Here's how the part is built. I have some questions about the finished solid (model axes, mm). Face numbers are marked on the shaded views. A direction names the side the tool comes from. Round coordinates to 2 decimals unless told otherwise and drop trailing zeros. Write each loop counter-clockwise with the first axis right and the second up, starting at its lowest first coordinate (ties: lowest second). Pieces come first, ordered by that corner, then holes. Notation, with made-up numbers: M 44,28.5 L 60,28.5 A32 cw 60,55.5 Z; hole C -13,-9.75 d4. An arc over 180 degrees is marked long. Use one line per item in the form item = value. Start each with the question number.
Q1. We'd pull the mould along Y, two halves only. Please class the marked faces 3, 4, 5 and 6: +Y half, -Y half, draft (parallel to the pull), parting line (faces both ways), or undercut.
Q2. I'm going to push flat-ended pins straight in: pin 1 Ø4 at (x, y) = (35.95, 15.88) entering from +Z; pin 2 Ø5 at (y, z) = (12, 2) entering from +X; pin 3 Ø4 at (y, z) = (14.5, -1.5) entering from -X; pin 4 Ø1.8 at (y, z) = (16.5, -1) entering from +X. Where does each tip first touch, or does it pass through?
Q3. I want a section at B-B on x = 20.5. List the corners of the cut face in (y, z) for me.
Q4. I want a section at C-C on z = 1.5. List the corners of the cut face in (x, y) for me (3 decimals).
Q5. I want a section at A-A on z = -1.5. List the corners of the cut face in (x, y) for me (3 decimals), and give its area (3 significant figures).
Q6. I need wall thicknesses on line 1 along Z through (x, y) = (11, 14); line 2 along X through (y, z) = (16, 1); line 3 along X through (y, z) = (16.5, 4). Which ranges of each line are inside material? Lowest first, please. Write a range as from..to.
Q7. For the marked faces 1 and 2, which set-ups out of +Z, -Z, +X, -X, +Y, -Y let a thin tool reach every point of the face, with its end or its side?
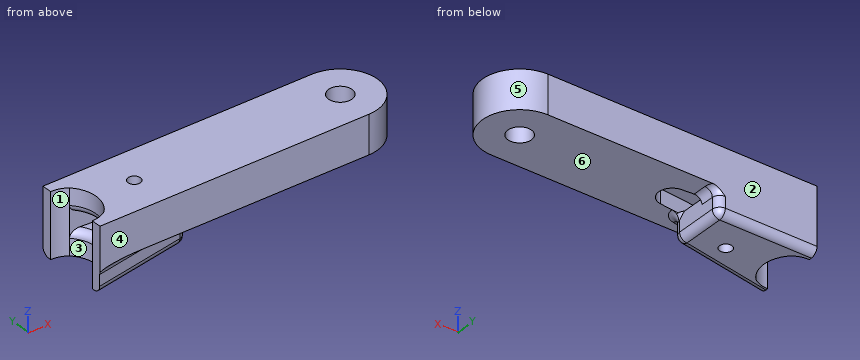
```python
from build123d import *

# Parameters (mm, degrees)
EXTRUDE_1_DEPTH     = 2.2
SKETCH_2_W          = 36.5
SKETCH_2_H          = 10.05
EXTRUDE_2_DEPTH     = 3.25
SKETCH_3_W          = 36.5
SKETCH_3_H          = 10.05
EXTRUDE_3_DEPTH     = 3.25
CUT_EXTRUDE_1_DEPTH = 30
SKETCH_6_R          = 5.025
EXTRUDE_4_DEPTH     = 8.7
SKETCH_8_R          = 1.675
SKETCH_8_R_2        = 0.84
CUT_EXTRUDE_3_DEPTH = 55
SKETCH_9_W          = 53.416465659
SKETCH_9_H          = 14.532409192
CUT_EXTRUDE_4_DEPTH = 3.5
SKETCH_10_R         = 1.6
CUT_EXTRUDE_5_DEPTH = 10
CUT_EXTRUDE_6_DEPTH = 3.5
FILLET_1_R          = 1
FILLET_2_R          = 1
FILLET_3_R          = 1


with BuildPart() as part:
    # 草图1 → 凸台-拉伸1 (new body)
    with BuildSketch(Plane.XY):
        with BuildLine():
            Line((1.539836705, 12.851012384), (15.55297303, 14.251012384))
            ThreePointArc((15.55297303, 14.251012384), (17.193415997, 16.063512384), (15.55297303, 17.876012384))
            Line((15.55297303, 17.876012384), (1.500532553, 18.901012384))
            ThreePointArc((1.500532553, 18.901012384), (0.527100583, 19.384612538), (-0.54702697, 19.551012384))
            Line((-0.54702697, 19.551012384), (-0.54702697, 20.901012384))
            Line((-0.54702697, 20.901012384), (19.51277613, 20.901012384))
            Line((19.51277613, 20.901012384), (35.95297303, 20.901012384))
            Line((35.95297303, 20.901012384), (35.95297303, 10.851012384))
            Line((35.95297303, 10.851012384), (-0.54702697, 10.851012384))
            Line((-0.54702697, 10.851012384), (-0.54702697, 12.201012384))
            ThreePointArc((-0.54702697, 12.201012384), (0.54584768, 12.367273294), (1.539836705, 12.851012384))
        make_face()
    extrude(amount=EXTRUDE_1_DEPTH)

    # 草图2 → 凸台-拉伸2 (add)
    with BuildSketch(Plane(origin=(0, 0, 0), x_dir=(-1, 0, 0), z_dir=(0, 0, -1))):
        with Locations((-17.70297303, 15.876012384)):
            Rectangle(SKETCH_2_W, SKETCH_2_H)
    extrude(amount=EXTRUDE_2_DEPTH)

    # 草图3 → 凸台-拉伸3 (add)
    with BuildSketch(Plane.XY.offset(2.2)):
        with Locations((17.70297303, 15.876012384)):
            Rectangle(SKETCH_3_W, SKETCH_3_H)
    extrude(amount=EXTRUDE_3_DEPTH)

    # 草图4 → 切除-拉伸1 (cut, symmetric)
    with BuildSketch(Plane.XY):
        with BuildLine():
            Line((-0.54702697, 19.551012384), (-2.235397712, 16.616091152))
            Line((-2.235397712, 16.616091152), (-1.110896638, 12.310548833))
            Line((-1.110896638, 12.310548833), (-0.54702697, 12.201012384))
            ThreePointArc((-0.54702697, 12.201012384), (0.54584768, 12.367273294), (1.539836705, 12.851012384))
            ThreePointArc((1.539836705, 12.851012384), (2.773180655, 15.88415254), (1.500532553, 18.901012384))
            ThreePointArc((1.500532553, 18.901012384), (0.527100583, 19.384612538), (-0.54702697, 19.551012384))
        make_face()
    extrude(amount=CUT_EXTRUDE_1_DEPTH, both=True, mode=Mode.SUBTRACT)

    # 草图6 → 凸台-拉伸4 (add)
    with BuildSketch(Plane(origin=(0, 0, -3.25), x_dir=(-1, 0, 0), z_dir=(0, 0, -1))):
        with Locations((-35.95297303, 15.876012384)):
            Circle(SKETCH_6_R)
    extrude(amount=-EXTRUDE_4_DEPTH)

    # 草图8 → 切除-拉伸3 (cut)
    with BuildSketch(Plane(origin=(0, 0, -3.25), x_dir=(-1, 0, 0), z_dir=(0, 0, -1))):
        with Locations((-49.45297303, 15.876012384)):
            Circle(SKETCH_8_R)
        with Locations(Location((-7.95297303, 15.856360308, 0), (0, 0, 180))):
            Circle(SKETCH_8_R_2)
    extrude(amount=-CUT_EXTRUDE_3_DEPTH, mode=Mode.SUBTRACT)

    # 草图9 → 切除-拉伸4 (cut)
    with BuildSketch(Plane(origin=(0, 0, -3.25), x_dir=(-1, 0, 0), z_dir=(0, 0, -1))):
        with Locations((-39.607660409, 15.039406696)):
            Rectangle(SKETCH_9_W, SKETCH_9_H)
    extrude(amount=-CUT_EXTRUDE_4_DEPTH, mode=Mode.SUBTRACT)

    # 草图10 → 切除-拉伸5 (cut)
    with BuildSketch(Plane.XY.offset(5.45)):
        with Locations((35.95297303, 15.876012384)):
            Circle(SKETCH_10_R)
    extrude(amount=-CUT_EXTRUDE_5_DEPTH, mode=Mode.SUBTRACT)

    # 草图11 → 切除-拉伸6 (cut)
    with BuildSketch(Plane(origin=(0, 0, -3.25), x_dir=(-1, 0, 0), z_dir=(0, 0, -1))):
        Polygon((-12.89942758, 13.294850275), (0.782882432, 10.851012384), (0, 8.730799831), (-15.448021962, 9.415407398), align=None)
    extrude(amount=-CUT_EXTRUDE_6_DEPTH, mode=Mode.SUBTRACT)

    # 圆角1
    fillet_1_edges = [part.edges().sort_by_distance(p)[0] for p in [
        (12.89942758, 20.901012384, -1.5),
        (12.89942758, 13.294850275, -1.5),
        (6.176200305, 12.093994751, -3.25),
        (12.89942758, 17.09793133, -3.25),
        (6.176200305, 20.901012384, -3.25),
    ]]
    fillet(fillet_1_edges, radius=FILLET_1_R)

    # 圆角2
    # the kernel refuses this fillet: 1 mm, written as the material it adds along each edge
    with BuildSketch(Plane(origin=(11.89942758, 14.132063378, 0.25), x_dir=(0.17583025935665297, -0.9844204995298362, 0), z_dir=(-0.9844204995298362, -0.17583025935665297, 0))) as fillet_2_piece_1_section:
        with BuildLine():
            CenterArc((1 + FILLET_2_R, -FILLET_2_R), FILLET_2_R, 90, 90)
            Line((1, -FILLET_2_R), (1, 0))
            Line((1, 0), (1 + FILLET_2_R, 0))
        make_face()
    fillet_2_piece_1 = revolve(axis=Axis((11.89942758, 14.132063378, 0.25), (0, 0, 1)), revolution_arc=214.681339144, mode=Mode.PRIVATE)
    fillet_2_piece_1 = split(fillet_2_piece_1, bisect_by=Plane(origin=(12.386461292, 13.934658048, 0.148039327), z_dir=(0.0994113635758644, -0.9950464214256476, 0)), keep=Keep.TOP, mode=Mode.PRIVATE)
    add(fillet_2_piece_1)
    with BuildSketch(Plane(origin=(11.89942758, 14.132063378, 0.25), x_dir=(0.17583025935665297, -0.9844204995298362, 0), z_dir=(-0.9844204995298362, -0.17583025935665297, 0))) as fillet_2_piece_2_section:
        with BuildLine():
            CenterArc((1 + FILLET_2_R, -FILLET_2_R), FILLET_2_R, 90, 90)
            Line((1, -FILLET_2_R), (1, 0))
            Line((1, 0), (1 + FILLET_2_R, 0))
        make_face()
    fillet_2_piece_2 = revolve(axis=Axis((11.89942758, 14.132063378, 0.25), (0, 0, 1)), revolution_arc=214.681339144, mode=Mode.PRIVATE)
    fillet_2_piece_2 = split(fillet_2_piece_2, bisect_by=Plane(origin=(12.896125684, 14.022775497, 0), z_dir=(0, 0, -1)), keep=Keep.TOP, mode=Mode.PRIVATE)
    add(fillet_2_piece_2)
    with BuildSketch(Plane(origin=(12.07525784, 13.147642879, 0.25), x_dir=(0, 0, -1), z_dir=(-0.984420499529836, -0.17583025935665386, 0))) as fillet_2_piece_3_section:
        with BuildLine():
            CenterArc((FILLET_2_R, FILLET_2_R), FILLET_2_R, 180, 90)
            Line((0, FILLET_2_R), (0, 0))
            Line((0, 0), (FILLET_2_R, 0))
        make_face()
    fillet_2_piece_3 = extrude(amount=15.32204588, mode=Mode.PRIVATE)
    fillet_2_piece_3 = split(fillet_2_piece_3, bisect_by=Plane(origin=(-0.54702697, 11.899303342, 0.017148227), z_dir=(1, 0, 0)), keep=Keep.TOP, mode=Mode.PRIVATE)
    fillet_2_piece_3 = split(fillet_2_piece_3, bisect_by=Plane(origin=(6.26358972, 10.851012384, 0.017148227), z_dir=(0, 1, 0)), keep=Keep.TOP, mode=Mode.PRIVATE)
    add(fillet_2_piece_3)
    with BuildSketch(Plane(origin=(11.89942758, 19.901012384, 0.25), x_dir=(-0.5976672776328282, -0.8017442392976477, 0), z_dir=(0.8017442392976477, -0.5976672776328282, 0))) as fillet_2_piece_4_section:
        with BuildLine():
            CenterArc((1 + FILLET_2_R, FILLET_2_R), FILLET_2_R, 180, 90)
            Line((1 + FILLET_2_R, 0), (1, 0))
            Line((1, 0), (1, FILLET_2_R))
        make_face()
    fillet_2_piece_4 = revolve(axis=Axis((11.89942758, 19.901012384, 0.25), (0, 0, -1)), revolution_arc=233.296989237, mode=Mode.PRIVATE)
    fillet_2_piece_4 = split(fillet_2_piece_4, bisect_by=Plane(origin=(12.649366525, 20.901012384, -0.061628308), z_dir=(0, -1, 0)), keep=Keep.TOP, mode=Mode.PRIVATE)
    add(fillet_2_piece_4)
    with BuildSketch(Plane(origin=(12.89942758, 15.56956482, 0.25), x_dir=(0, 0, -1), z_dir=(0, 1, 0))) as fillet_2_piece_5_section:
        with BuildLine():
            CenterArc((FILLET_2_R, -FILLET_2_R), FILLET_2_R, 90, 90)
            Line((0, -FILLET_2_R), (0, 0))
            Line((0, 0), (FILLET_2_R, 0))
        make_face()
    fillet_2_piece_5 = extrude(amount=4.331447564, mode=Mode.PRIVATE)
    fillet_2_piece_5 = split(fillet_2_piece_5, bisect_by=Plane(origin=(12.930705697, 18.067283361, -0.180311335), z_dir=(0.0727477998867751, 0.9973503685323598, 0)), keep=Keep.TOP, mode=Mode.PRIVATE)
    add(fillet_2_piece_5)

    # 圆角3
    fillet_3_edges = [part.edges().sort_by_distance(p)[0] for p in [
        (2.773180655, 15.88415254, 0),
        (2.773180655, 15.88415254, 2.2),
    ]]
    fillet(fillet_3_edges, radius=FILLET_3_R)


solid = part.part
```
Reported:
q1.face_3 = undercut
q1.face_4 = -Y half
q1.face_5 = parting line
q1.face_6 = draft
q2.pin_1 = 5.45
q2.pin_2 = 40.79
q2.pin_3 = 0.9
q2.pin_4 = 12.9
q3.outline = M 10.85,0.25 L 20.9,0.25 L 20.9,5.45 L 10.85,5.45 Z
q4.outline = M -0.547,10.851 L 35.953,10.851 A5.025 ccw 35.953,20.901 L -0.547,20.901 L -0.547,19.551 A3.55 cw 1.501,18.901 L 15.553,17.876 A1.822 cw 15.553,14.251 L 1.54,12.851 A3.675 cw -0.547,12.201 Z; hole C 35.953,15.876 d3.2
q5.outline = M -0.547,10.893 L 12.075,13.148 A1 ccw 12.899,14.132 L 12.899,19.901 A1 ccw 11.899,20.901 L -0.547,20.901 L -0.547,19.551 A3.55 cw 1.501,18.901 A4.278 cw 1.54,12.851 A3.675 cw -0.547,12.201 Z; hole C 7.953,15.856 d1.68
q5.area = 96.3 mm^2
q6.line_1 = -3.25..0, 2.2..5.45
q6.line_2 = 17.19..34.36, 37.55..40.98
q6.line_3 = 2.72..7.41, 8.49..34.48, 37.43..40.94
q7.face_1 = +Z, -Z, -X
q7.face_2 = +Z, -Z, +X, -X, +Y
